```python
from build123d import *

# Parameters (mm, degrees)
EXTRUDE_1_DEPTH = 40


with BuildPart() as part:
    # Эскиз1 → Бобышка-Вытянуть1 (new body)
    with BuildSketch(Plane.XY):
        with BuildLine():
            Line((0, 0), (0, -5))
            Line((0, -5), (-0.235052359, -5))
            Line((-0.235052359, -5), (-0.235052359, -6.077530645))
            Line((-0.235052359, -6.077530645), (1.580879478, -10.300026718))
            Line((1.580879478, -10.300026718), (2.299876794, -10.300026718))
            Line((2.299876794, -10.300026718), (2.299876794, -8.688248945))
            Line((2.299876794, -8.688248945), (5.338733825, -6.749380382))
            Line((5.338733825, -6.749380382), (5.338733825, -6.130118817))
            ThreePointArc((5.338733825, -6.130118817), (5.151167457, -5.800618872), (4.772085378, -5.793681018))
            Line((4.772085378, -5.793681018), (2.085504308, -7.258574696))
            Line((2.085504308, -7.258574696), (2.085504308, -4.45645656))
            Line((2.085504308, -4.45645656), (5.980110004, -2.374221663))
            Line((5.980110004, -2.374221663), (5.980110004, -1.617236279))
            ThreePointArc((5.980110004, -1.617236279), (5.788765805, -1.262133881), (5.386956071, -1.226647924))
            Line((5.386956071, -1.226647924), (2.15420838, -2.616927359))
            Line((2.15420838, -2.616927359), (2.15420838, 0.497930702))
            Line((2.15420838, 0.497930702), (5.024831948, 3.373619708))
            Line((5.024831948, 3.373619708), (4.333601466, 4.294416481))
            ThreePointArc((4.333601466, 4.294416481), (1.705007112, 2.626935837), (-1.152317838, 1.391745925))
            Line((-1.152317838, 1.391745925), (-1.152317838, 0))
            Line((-1.152317838, 0), (0, 0))
        make_face()
    extrude(amount=EXTRUDE_1_DEPTH)


solid = part.part
```
Read the model definition and answer for the solid it produces. Units are mm, in the model's axes. A direction names the side the tool comes from. Coordinates: 2 decimals unless noted, no trailing zeros. Write each loop counter-clockwise with the first axis right and the second up, starting at its lowest first coordinate (ties: lowest second). Pieces come first, ordered by that corner, then holes. Notation, with made-up numbers: (37.5, 36) - (63.5, 36) arc R17 cw to (63.5, 58) - close; hole circle Ø9 at (80.25, 39). An arc over 180 degrees is marked (long way). Answer as a JSON object with one key per item and string values. Group by question number.
1. A cutting plane is placed at B-B (z = 19.5). Determine the outline of the cut face in (x, y).
2. Each of these flat-tipped pins is pushed along its axis until it touches: P1, Ø1.8, axis at y = -9.5, z = 13, coming from the +X side; P2, Ø1.4, axis at y = -6, z = 29, coming from the +X side; P3, Ø2, axis at x = 3, y = -8.5, coming from the -Z side; P4, Ø1.5, axis at y = 2.5, z = 26, coming from the +X side. Where does it stop, or does it pass through?
3. Consider L1, parallel to Y at x = 4, z = 10; L2, parallel to Y at x = 2.5, z = 22.5; L3, parallel to X at y = -5.5, z = 7.5. Determine where each line is inside the solid, lowest interval first. Write a range as [from, to].
4. Which of the six approach directions +Z, -Z, +X, -X, +Y, -Y give full straight-line access (tool end or side, diameter ignored) to faces 4 (the flat face through (3.448, -6.516, 19.72)), 5 (the flat face through (2.3, -10, 20)), 6 (the flat face through (-0.235, -5.5, 19.7)), 7 (the flat face through (0, -2, 20)), 8 (the flat face through (3.569, 1.916, 19.72))?
5. A cutting plane is placed at C-C (y = 1). Determine the outline of the cut face in (x, z), plus the area to 3 significant figures.
6. A cutting plane is placed at A-A (x = 3.5). Determine the outline of the cut face in (y, z), plus the area to 3 significant figures.
7. The mould has two halves that part along Y. Classify faces 1 (the flat face through (3.8, -7.73, 19.72)), 2 (the cylindrical face through (1.744, 2.647, 19.72)), 3 (the flat face through (4.006, -3.43, 19.72)): +Y half, -Y half, draft (parallel to the pull), parting line (faces both ways), or undercut.
8. A cutting plane is placed at D-D (y = -3.75). Determine the outline of the cut face in (x, z), plus the area to 3 significant figures.
Worked out:
{
 "1": {"outline": "(-1.15, 0) - (0, 0) - (0, -5) - (-0.24, -5) - (-0.24, -6.08) - (1.58, -10.3) - (2.3, -10.3) - (2.3, -8.69) - (5.34, -6.75) - (5.34, -6.13) arc R0.38 ccw to (4.77, -5.79) - (2.09, -7.26) - (2.09, -4.46) - (5.98, -2.37) - (5.98, -1.62) arc R0.43 ccw to (5.39, -1.23) - (2.15, -2.62) - (2.15, 0.5) - (5.02, 3.37) - (4.33, 4.29) arc R19.81 cw to (-1.15, 1.39) - close"},
 "2": {"P1": "stops at x = 2.44", "P2": "stops at x = 5.34", "P3": "stops at z = 0", "P4": "stops at x = 4.9"},
 "3": {"L1": "y = [-7.6, -6.21], [-3.43, -1.82], [2.35, 4.05]", "L2": "y = [-8.56, -7.03], [-4.23, -2.47], [0.84, 3.07]", "L3": "x = [-0.24, 2.09]"},
 "4": {"face 4": "+Z, -Z", "face 5": "+Z, -Z, +X, -Y", "face 6": "+Z, -Z, -X, -Y", "face 7": "+Z, -Z, -X", "face 8": "+Z, -Z, +X"},
 "5": {"outline": "(-1.15, 0) - (2.66, 0) - (2.66, 40) - (-1.15, 40) - close", "area": "152 mm²"},
 "6": {"outline": "(-7.92, 0) - (-6.49, 0) - (-6.49, 40) - (-7.92, 40) - close; (-3.7, 0) - (-2.04, 0) - (-2.04, 40) - (-3.7, 40) - close; (1.85, 0) - (3.7, 0) - (3.7, 40) - (1.85, 40) - close", "area": "198 mm²"},
 "7": {"face 1": "-Y half", "face 2": "+Y half", "face 3": "undercut"},
 "8": {"outline": "(0, 0) - (3.41, 0) - (3.41, 40) - (0, 40) - close", "area": "136 mm²"}
}
